Geometry check sheet. Reference: the model listing, model coordinates, mm. A direction names the side the tool comes from. Round coordinates to 2 decimals unless told otherwise and drop trailing zeros. Order: outer loops, then holes, each group sorted by start corner. A loop starts at its lowest first (then second) coordinate and runs counter-clockwise, first axis right, second up. Notation, with made-up numbers: (-38.5, 55.25) - (10.5, 55.25) arc R34 cw to (10.5, 87.25) - close; hole circle Ø8 at (13, -16). An arc over 180 degrees is marked (long way). Return JSON: item names as keys, results as strings. Group by question number.
Q1. Draft check along Z on faces 1 (the flat face through (2, 3.175, -1)), 2 (the cylindrical face through (-82.55, 1.57, 24.27)). Enter one of: pulls with the +Z half, pulls with the -Z half, needs draft (parallel to the pull), parting line crosses it, or undercut.
Q2. Gauge pin test, flat ends, axial feed: pin 1 Ø1 at (x, y) = (-104.5, 1.5) entering from -Z; pin 2 Ø1 at (y, z) = (1.59, 0) entering from -X; pin 3 Ø10 at (x, z) = (-48.5, -20.5) entering from +Y (3 decimals); pin 4 Ø1.4 at (x, y) = (105, 2) entering from +Z. Record the tip position at first contact, or that the pin passes through.
Q3. Material ranges on line 1 along Z through (x, y) = (-29, 0.35); line 2 along Y through (x, z) = (56, 0) (1 decimal); line 3 along X through (y, z) = (0.5, -23.5), recorded low to high.
Q4. Sectioned sample at B-B, the plane x = -38. Record the cut outline in (y, z) (1 decimal), then the cut area to 3 significant figures.
Q5. Sectioned sample at A-A, the plane z = -20. Record the cut outline in (x, y) (3 decimals), then the cut area to 3 significant figures.
Q6. Tool access check on faces 3 (the cylindrical face through (-19.05, 1.57, -23.99)), 4 (the flat face through (2, 0, -1)). Record the directions out of +Z, -Z, +X, -X, +Y, -Y that give a thin tool (end or side, any length) a straight path to the whole face; none if there is none.
```python
from build123d import *

# Parameters (mm, degrees)
BOSS_EXTRUDE1_DEPTH = 3.175
FILLET1_R           = 2.54
SKETCH3_R           = 0.635
CUT_EXTRUDE1_DEPTH  = 213.785648071


with BuildPart() as part:
    # Sketch1 → Boss-Extrude1 (new body)
    with BuildSketch(Plane(origin=(0, 0, 0), x_dir=(1, 0, 0), z_dir=(0, 1, 0))):
        Polygon((-101.6, 36.83), (101.6, 36.83), (101.6, 26.67), (107.95, 26.67), (107.95, 10.16), (101.6, 10.16), (101.6, -10.16), (107.95, -10.16), (107.95, -26.67), (101.6, -26.67), (101.6, -36.83), (-101.6, -36.83), (-101.6, -26.67), (-107.95, -26.67), (-107.95, -10.16), (-101.6, -10.16), (-101.6, 10.16), (-107.95, 10.16), (-107.95, 26.67), (-101.6, 26.67), align=None)
        with BuildLine():
            Line((-76.2, -17.78), (-25.4, -17.78))
            ThreePointArc((-25.4, -17.78), (-19.05, -24.13), (-25.4, -30.48))
            Line((-25.4, -30.48), (-76.2, -30.48))
            ThreePointArc((-76.2, -30.48), (-82.55, -24.13), (-76.2, -17.78))
        make_face(mode=Mode.SUBTRACT)
        with BuildLine():
            Line((-76.2, 17.78), (-25.4, 17.78))
            ThreePointArc((-25.4, 17.78), (-19.05, 24.13), (-25.4, 30.48))
            Line((-25.4, 30.48), (-76.2, 30.48))
            ThreePointArc((-76.2, 30.48), (-82.55, 24.13), (-76.2, 17.78))
        make_face(mode=Mode.SUBTRACT)
    extrude(amount=BOSS_EXTRUDE1_DEPTH)

    # Fillet1
    fillet1_edges = [part.edges().sort_by_distance(p)[0] for p in [
        (101.6, 1.5875, 36.83),
        (-101.6, 1.5875, 36.83),
        (-101.6, 1.5875, 26.67),
        (-107.95, 1.5875, 26.67),
        (-107.95, 1.5875, 10.16),
        (-101.6, 1.5875, 10.16),
        (-101.6, 1.5875, -10.16),
        (-107.95, 1.5875, -10.16),
        (-107.95, 1.5875, -26.67),
        (-101.6, 1.5875, -26.67),
        (-101.6, 1.5875, -36.83),
        (101.6, 1.5875, -36.83),
        (101.6, 1.5875, -26.67),
        (107.95, 1.5875, -26.67),
        (107.95, 1.5875, -10.16),
        (101.6, 1.5875, -10.16),
        (101.6, 1.5875, 10.16),
        (107.95, 1.5875, 10.16),
        (107.95, 1.5875, 26.67),
        (101.6, 1.5875, 26.67),
    ]]
    fillet(fillet1_edges, radius=FILLET1_R)

    # Sketch3 → Cut-Extrude1 (cut, through all)
    with BuildSketch(Plane.ZY.offset(101.6)):
        with Locations((0, 1.5875)):
            Circle(SKETCH3_R)
    extrude(amount=-CUT_EXTRUDE1_DEPTH, mode=Mode.SUBTRACT)


solid = part.part
```
Reply:
{
 "1": {"face 1": "needs draft", "face 2": "undercut"},
 "2": {"pin 1": "z = -26.67", "pin 2": "through", "pin 3": "y = 3.175", "pin 4": "z = 26.67"},
 "3": {"line 1": "-36.83 to -30.48, -17.78 to 17.78, 30.48 to 36.83", "line 2": "0 to 1, 2.2 to 3.2", "line 3": "-107.95 to -82.52, -19.08 to 107.95"},
 "4": {"outline": "(0, -36.8) - (3.2, -36.8) - (3.2, -30.5) - (0, -30.5) - close; (0, -17.8) - (3.2, -17.8) - (3.2, 17.8) - (0, 17.8) - close; (0, 30.5) - (3.2, 30.5) - (3.2, 36.8) - (0, 36.8) - close; hole circle Ø1.3 at (1.6, 0)", "area": "152 mm^2"},
 "5": {"outline": "(-107.95, 0) - (-81.023, 0) - (-81.023, 3.175) - (-107.95, 3.175) - close; (-20.577, 0) - (107.95, 0) - (107.95, 3.175) - (-20.577, 3.175) - close", "area": "494 mm^2"},
 "6": {"face 3": "+Y, -Y", "face 4": "+Z, -Z, +X, -X, -Y"}
}
